from build123d import *

# Parameters (mm, degrees)
F0_W     = 50.8
F0_H     = 6.35
F1_DEPTH = 177.8
F2_W     = 25.4
F2_H     = 13.97
F2_H_2   = 11.684
F2_W_2   = 31.75
F2_H_3   = 25.4
F3_DEPTH = 25.4


with BuildPart() as f1:
    # F0 (on Right) → F1 (new body)
    with BuildSketch(Plane.YZ):
        with Locations((-14.505542, 1.499517)):
            Rectangle(F0_W, F0_H)
        Polygon((10.894458, 23.724517), (-39.905542, 4.674517), (10.894458, 4.674517), align=None)
        Polygon((-39.905542, -1.675483), (-39.905542, 4.674517), (-39.905542, 11.024517), (-43.080542, 11.024517), (-43.080542, -1.675483), align=None)
    extrude(amount=F1_DEPTH)

    # F2 (on face) → F3 (cut)
    with BuildSketch(Plane(origin=(0, -6.456689, 17.217837), x_dir=(1, 0, 0), z_dir=(0, -0.351123, 0.936329))):
        Polygon((101.6, -29.551553), (114.3, -29.551553), (114.3, -14.311553), (88.9, -14.311553), (88.9, -29.551553), align=None)
        with Locations((63.5, -22.566553)):
            Rectangle(F2_W, F2_H)
        with Locations((25.4, -23.709553)):
            Rectangle(F2_W, F2_H_2)
        with Locations((142.875, -16.851553)):
            Rectangle(F2_W_2, F2_H_3)
    extrude(amount=-F3_DEPTH, mode=Mode.SUBTRACT)


solid = f1.part
Read the model definition and answer for the solid it produces. Units are mm, in the model's axes. A direction names the side the tool comes from. Coordinates: 2 decimals unless noted, no trailing zeros. Loops run counter-clockwise (first coordinate to the right, second up) from the corner with the lowest first, then second, coordinate; pieces in that order, holes last.
Q1. The part is cut by section B-B on z = 0.25. Write down the section's boundary in (x, y).
Q2. Which of the six approach directions +Z, -Z, +X, -X, +Y, -Y give full straight-line access (tool end or side, diameter ignored) to faces 4 (the face through (25.22, -32.55, 2.64)), 5 (the face through (88, -39.906, 8)), 6 (the face through (142.65, -7.12, 7.16)), 7 (the face through (38.1, -27, 4))?
Q3. Each of these flat-tipped pins is pushed along its axis until it touches: pin 1 Ø2.5 at (x, y) = (111.5, -42) entering from +Z; pin 2 Ø1 at (x, y) = (112, -19.5) entering from +Z. Where does it stop, or does it pass through?
Q4. The mould has two halves that part along X. Classify faces 1 (the face through (88, 10.894, 11)), 2 (the face through (0, -10, 8)), 3 (the face through (25.222, -20.854, 4.723)): +X half, -X half, draft (parallel to the pull), parting line (faces both ways), or undercut.
Q5. Consider probe 1 along X at (y, z) = (-21, 6); probe 2 along X at (y, z) = (-7, 2); probe 3 along Z at (x, y) = (26, -8.5). Determine where each line is inside the solid, lowest interval first.
Q6. The part is cut by section A-A on x = 136. Write down the section's boundary in (y, z).
Q7. The part is cut by section C-C on x = 57.5. Write down the section's boundary in (y, z).
Q8. The part is cut by section D-D on y = -27. Write down the section's boundary in (x, z).
Results below:
1. outline: (0, -43.08) - (177.8, -43.08) - (177.8, 10.89) - (0, 10.89) - close; hole (12.7, -31.65) - (38.1, -31.65) - (38.1, -19.18) - (12.7, -19.18) - close; hole (50.8, -31.65) - (76.2, -31.65) - (76.2, -16.73) - (50.8, -16.73) - close; hole (88.9, -31.65) - (114.3, -31.65) - (114.3, -15.38) - (88.9, -15.38) - close; hole (127, -31.65) - (158.75, -31.65) - (158.75, -4.53) - (127, -4.53) - close
2. face 4: +Z
2. face 5: +Z, +X, -X
2. face 6: -Z
2. face 7: none
3. pin 1: stops at z = 11.02
3. pin 2: stops at z = 12.51
4. face 1: draft
4. face 2: -X half
4. face 3: undercut
5. probe 1: x = 0 to 50.8, 76.2 to 88.9, 114.3 to 127, 158.75 to 177.8
5. probe 2: x = 0 to 127, 158.75 to 177.8
5. probe 3: z = -1.68 to 16.45
6. outline: (-43.08, -1.68) - (-30.93, -1.68) - (-34.13, 6.84) - (-39.91, 4.67) - (-39.91, 11.02) - (-43.08, 11.02) - close; (-10.34, 15.76) - (-3.81, -1.68) - (10.89, -1.68) - (10.89, 23.72) - close
7. outline: (-43.08, -1.68) - (-30.93, -1.68) - (-34.13, 6.84) - (-39.91, 4.67) - (-39.91, 11.02) - (-43.08, 11.02) - close; (-21.05, 11.75) - (-16.01, -1.68) - (10.89, -1.68) - (10.89, 23.72) - close
8. outline: (0, -1.68) - (12.7, -1.68) - (12.7, 9.51) - (0, 9.51) - close; (38.1, -1.68) - (50.8, -1.68) - (50.8, 9.51) - (38.1, 9.51) - close; (76.2, -1.68) - (88.9, -1.68) - (88.9, 9.51) - (76.2, 9.51) - close; (114.3, -1.68) - (127, -1.68) - (127, 9.51) - (114.3, 9.51) - close; (158.75, -1.68) - (177.8, -1.68) - (177.8, 9.51) - (158.75, 9.51) - close
